Source: CAD feature listing. Evaluate the final solid. Frame: model axes, mm. A direction names the side the tool comes from. Coordinates: 2 decimals unless noted, no trailing zeros. Write each loop counter-clockwise with the first axis right and the second up, starting at its lowest first coordinate (ties: lowest second). Pieces come first, ordered by that corner, then holes. Notation, with made-up numbers: (20.25, -20) - (64.25, -20) arc R16 ccw to (64.25, 6) - close; hole circle Ø3 at (27.25, -23.5). An arc over 180 degrees is marked (long way). One line per question, with ' | ' between items.
from build123d import *

# Parameters (mm, degrees)
F0_R     = 5.25
F0_R_2   = 3.25
F0_R_3   = 2.75
F1_DEPTH = 4
F2_R     = 8


with BuildPart() as f1:
    # F0 (on Top) → F1 (new body)
    with BuildSketch(Plane.XY):
        with BuildLine():
            Line((46.978489, 11.25), (0, 11.25))
            ThreePointArc((0, 11.25), (-11.224612, -0.755377), (1.507345, -11.148561))
            Line((1.507345, -11.148561), (42.089501, -5.661638))
            Line((42.089501, -5.661638), (81.481345, -10.149772))
            ThreePointArc((81.481345, -10.149772), (88.62135, -4.803506), (83.701447, 2.636708))
            Line((83.701447, 2.636708), (46.978489, 11.25))
        make_face()
        Circle(F0_R, mode=Mode.SUBTRACT)
        with Locations((82.217166, -3.691555)):
            Circle(F0_R_2, mode=Mode.SUBTRACT)
        with Locations((42.891439, 3.053603)):
            Circle(F0_R_3, mode=Mode.SUBTRACT)
    extrude(amount=F1_DEPTH)

    # F2
    f2_edges = [f1.edges().sort_by_distance(p)[0] for p in [
        (42.089501, -5.661638, 2),
        (46.978489, 11.25, 2),
    ]]
    fillet(f2_edges, radius=F2_R)


solid = f1.part
Item 1: Mould query, pull axis X, two halves, no side actions, for faces 3 (the face through (23, 11.25, 2)), 4 (the face through (62.01, -7.93, 1.97)), 5 (the face through (46.96, 11.2, 2.03)). Classes: pulls with the +X half, pulls with the -X half, needs draft (parallel to the pull), parting line crosses it, or undercut.
Check sheet entries:
face 3: needs draft | face 4: undercut | face 5: pulls with the +X half
Item 2: Cut plane B-B on z = 2.1. Return loops of the section in (x, y), and give its area (3 significant figures).
Check sheet entries:
outline: (0, 11.25) arc R11.25 ccw (long way) to (1.51, -11.15) - (41.1, -5.8) arc R8 cw to (43.08, -5.77) - (81.48, -10.15) arc R6.5 ccw to (83.7, 2.64) - (47.88, 11.04) arc R8 ccw to (46.05, 11.25) - close; hole circle Ø10.5 at (0, 0); hole circle Ø5.5 at (42.89, 3.05); hole circle Ø6.5 at (82.22, -3.69) | area: 1,580 mm²
Item 3: Ray query, line 1 along Y through (x, z) = (0, 1.9); line 2 along X through (y, z) = (-3, 1.2); line 3 along Y through (x, z) = (35, 1.7). Return the intervals inside material, ascending. Write a range as [from, to].
Check sheet entries:
line 1: [-11.25, -5.25], [5.25, 11.25] | line 2: [-10.84, -4.31], [4.31, 79.04], [85.39, 88.68] | line 3: [-6.62, 11.25]
Item 4: Cut plane C-C on x = 66. Return loops of the section in (y, z).
Check sheet entries:
outline: (-8.39, 0) - (6.79, 0) - (6.79, 4) - (-8.39, 4) - close
Item 5: Access query for faces 1 (the face through (21.03, -8.51, 1.97)), 2 (the face through (38, 0, 4)). Directions: +Z, -Z, +X, -X, +Y, -Y. A direction counts if a zero-diameter tool reaches every point of the face in a straight line with its end or side. Return the directions, or none.
Check sheet entries:
face 1: +Z, -Z, -Y | face 2: +Z, +X, -X, +Y, -Y
Item 6: Cut plane A-A on y = -2. Return loops of the section in (x, z).
Check sheet entries:
outline: (-11.07, 0) - (-4.85, 0) - (-4.85, 4) - (-11.07, 4) - close; (4.85, 0) - (79.44, 0) - (79.44, 4) - (4.85, 4) - close; (84.99, 0) - (88.49, 0) - (88.49, 4) - (84.99, 4) - close
